Verification items for the finished model (mm, model axes). Face numbers are marked on the shaded views. A direction names the side the tool comes from. Round coordinates to 2 decimals unless told otherwise and drop trailing zeros. Order: outer loops, then holes, each group sorted by start corner. A loop starts at its lowest first (then second) coordinate and runs counter-clockwise, first axis right, second up. Notation, with made-up numbers: (34.5, -12) -> (85.5, -12) arc R4 ccw to (85.5, -8) -> close; hole circle Ø8 at (-9.75, 24.5). An arc over 180 degrees is marked (long way). Return JSON: item names as keys, results as strings. Group by question number.
1) Section check C-C on x = 12. Enter the section's corners in (y, z), plus the area to 3 significant figures.
2) Section check D-D on z = -19.5. Enter the section's corners in (x, y), plus the area to 3 significant figures.
3) Section check A-A on y = 0. Enter the section's corners in (x, z) (3 decimals).
4) Tool access check on the marked faces 1 and 2. Record the directions out of +Z, -Z, +X, -X, +Y, -Y that give a thin tool (end or side, any length) a straight path to the whole face; none if there is none.
5) Scan lines: L1, parallel to X at y = -29, z = -25; L2, parallel to Y at x = 0, z = 2.4 (3 decimals); L3, parallel to Y at x = 3.5, z = -33.5. Record each from-to range of solid material in increasing order.
6) Depth check by flat-ended pin: pin 1 (8 mm diameter, centred on x = 3, y = 21.5, fed in from -Z); pin 2 (5 mm diameter, centred on x = 18, z = -25, fed in from +Y); pin 3 (4 mm diameter, centred on x = 8, y = -14.5, fed in from +Z). Enter the tip coordinate at first touch or a pass-through.
7) Section check B-B on z = -25. Enter the section's corners in (x, y).
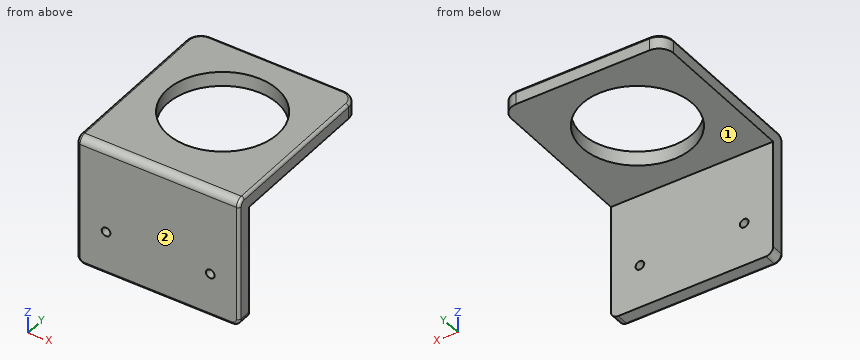
```python
from build123d import *

# Parameters (mm, degrees)
ESQUISSE1_R             = 19.075
BOSS_EXTRU_2_DEPTH      = 5
ESQUISSE2_W             = 56
ESQUISSE2_H             = 5
BOSS_EXTRU_3_DEPTH      = 5
ESQUISSE3_W             = 56
ESQUISSE3_H             = 5
BOSS_EXTRU_4_DEPTH      = 50
CONG_1_R                = 2.5
ESQUISSE5_R             = 1.5
ENL_V_MAT_EXTRU_2_DEPTH = 5
ESQUISSE6_W             = 56
ESQUISSE6_H             = 5
ENL_V_MAT_EXTRU_3_DEPTH = 10
CONG_2_R                = 2.5
CONG_3_R                = 1


with BuildPart() as part:
    # Esquisse1 → Boss.-Extru.2 (new body)
    with BuildSketch(Plane.XY):
        with BuildLine():
            Line((-23, 28), (23, 28))
            ThreePointArc((23, 28), (26.535533906, 26.535533906), (28, 23))
            Line((28, 23), (28, -28))
            Line((28, -28), (-28, -28))
            Line((-28, -28), (-28, 23))
            ThreePointArc((-28, 23), (-26.535533906, 26.535533906), (-23, 28))
        make_face()
        Circle(ESQUISSE1_R, mode=Mode.SUBTRACT)
    extrude(amount=BOSS_EXTRU_2_DEPTH)

    # Esquisse2 → Boss.-Extru.3 (add)
    with BuildSketch(Plane.XZ.offset(28)):
        with Locations((0, 2.5)):
            Rectangle(ESQUISSE2_W, ESQUISSE2_H)
    extrude(amount=BOSS_EXTRU_3_DEPTH)

    # Esquisse3 → Boss.-Extru.4 (add)
    with BuildSketch(Plane(origin=(0, 0, 0), x_dir=(-1, 0, 0), z_dir=(0, 0, -1))):
        with Locations((0, -30.5)):
            Rectangle(ESQUISSE3_W, ESQUISSE3_H)
    extrude(amount=BOSS_EXTRU_4_DEPTH)

    # Congé1
    cong_1_edges = [part.edges().sort_by_distance(p)[0] for p in [
        (0, -33, 5),
    ]]
    fillet(cong_1_edges, radius=CONG_1_R)

    # Esquisse5 → Enlèv. mat.-Extru.2 (cut)
    with BuildSketch(Plane(origin=(0, -28, 0), x_dir=(1, 0, 0), z_dir=(0, 1, 0))):
        with Locations(Location((-18, 25, 0), (0, 0, 270))):
            Circle(ESQUISSE5_R)
        with Locations(Location((18, 25, 0), (0, 0, 90))):
            Circle(ESQUISSE5_R)
    extrude(amount=-ENL_V_MAT_EXTRU_2_DEPTH, mode=Mode.SUBTRACT)

    # Esquisse6 → Enlèv. mat.-Extru.3 (cut)
    with BuildSketch(Plane(origin=(0, 0, -50), x_dir=(-1, 0, 0), z_dir=(0, 0, -1))):
        with Locations((0, -30.5)):
            Rectangle(ESQUISSE6_W, ESQUISSE6_H)
    extrude(amount=-ENL_V_MAT_EXTRU_3_DEPTH, mode=Mode.SUBTRACT)

    # Congé2
    cong_2_edges = [part.edges().sort_by_distance(p)[0] for p in [
        (28, -30.5, -40),
        (-28, -30.5, -40),
    ]]
    fillet(cong_2_edges, radius=CONG_2_R)

    # Congé3
    cong_3_edges = [part.edges().sort_by_distance(p)[0] for p in [
        (0, 28, 5),
        (-26.535533906, 26.535533906, 5),
        (-28, -3.75, 5),
        (-28, -33, -17.5),
        (-28, -32.267766953, 4.267766953),
        (28, -3.75, 5),
        (28, -32.267766953, 4.267766953),
        (0, -33, -40),
        (26.535533906, 26.535533906, 5),
        (28, -33, -17.5),
        (27.267766953, -33, -39.267766953),
        (-27.267766953, -33, -39.267766953),
    ]]
    fillet(cong_3_edges, radius=CONG_3_R)


solid = part.part
```
Check result:
{
 "1": {"outline": "(-33, -39) arc R1 ccw to (-32, -40) -> (-28, -40) -> (-28, 0) -> (-14.83, 0) -> (-14.83, 5) -> (-30.5, 5) arc R2.5 ccw to (-33, 2.5) -> close; (14.83, 0) -> (28, 0) -> (28, 4) arc R1 ccw to (27, 5) -> (14.83, 5) -> close", "area": "355 mm^2"},
 "2": {"outline": "(-28, -32) arc R1 ccw to (-27, -33) -> (27, -33) arc R1 ccw to (28, -32) -> (28, -28) -> (-28, -28) -> close", "area": "280 mm^2"},
 "3": {"outline": "(-28, 0) -> (-19.075, 0) -> (-19.075, 5) -> (-27, 5) arc R1 ccw to (-28, 4) -> close; (19.075, 0) -> (28, 0) -> (28, 4) arc R1 ccw to (27, 5) -> (19.075, 5) -> close"},
 "4": {"face 1": "-Z, +X, -X, +Y", "face 2": "+Z, -Z, +X, -X, -Y"},
 "5": {"L1": "-28 to -19.5, -16.5 to 16.5, 19.5 to 28", "L2": "-33 to -19.075, 19.075 to 28", "L3": "-33 to -28"},
 "6": {"pin 1": "z = 0", "pin 2": "y = -28", "pin 3": "through"},
 "7": {"outline": "(-28, -32) arc R1 ccw to (-27, -33) -> (-19.5, -33) -> (-19.5, -28) -> (-28, -28) -> close; (-16.5, -33) -> (16.5, -33) -> (16.5, -28) -> (-16.5, -28) -> close; (19.5, -33) -> (27, -33) arc R1 ccw to (28, -32) -> (28, -28) -> (19.5, -28) -> close"}
}
